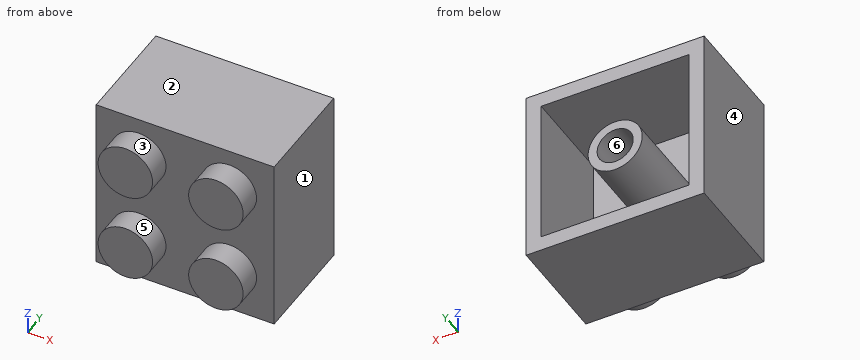
from build123d import *

# Parameters (mm, degrees)
F0_W     = 15.78
F0_H     = 15.78
F0_R     = 2.415
F1_DEPTH = 9.6
F2_DEPTH = 11.76
F3_W     = 13.12
F3_H     = 13.12
F3_R     = 2.415
F3_R_2   = 2.4
F4_DEPTH = 8.38
F3_R_3   = 1.6
F5_DEPTH = 8.38


with BuildPart() as f1:
    # F0 (on Front) → F1 (new body)
    with BuildSketch(Plane.XZ):
        Rectangle(F0_W, F0_H)
        with Locations((-4.115, -3.915)):
            Circle(F0_R, mode=Mode.SUBTRACT)
        with Locations((3.915, -3.915)):
            Circle(F0_R, mode=Mode.SUBTRACT)
        with Locations((-4.115, 4.115)):
            Circle(F0_R, mode=Mode.SUBTRACT)
        with Locations((3.915, 4.115)):
            Circle(F0_R, mode=Mode.SUBTRACT)
    extrude(amount=F1_DEPTH)

    # F0 (on Front) → F2 (join)
    with BuildSketch(Plane.XZ):
        with Locations((-4.115, 4.115)):
            Circle(F0_R)
        with Locations((3.915, 4.115)):
            Circle(F0_R)
        with Locations((-4.115, -3.915)):
            Circle(F0_R)
        with Locations((3.915, -3.915)):
            Circle(F0_R)
    extrude(amount=F2_DEPTH)

    # F3 (on face) → F4 (cut)
    with BuildSketch(Plane.XZ):
        Rectangle(F3_W, F3_H)
        with Locations((-4.115, -3.915)):
            Circle(F3_R, mode=Mode.SUBTRACT)
        with Locations((3.915, -3.915)):
            Circle(F3_R, mode=Mode.SUBTRACT)
        with Locations((-4.115, 4.115)):
            Circle(F3_R, mode=Mode.SUBTRACT)
        Circle(F3_R_2, mode=Mode.SUBTRACT)
        with Locations((3.915, 4.115)):
            Circle(F3_R, mode=Mode.SUBTRACT)
    extrude(amount=F4_DEPTH, mode=Mode.SUBTRACT)

    # F0 (on Front) + F3 (on face) → F5 (cut)
    with BuildSketch(Plane.XZ):
        with Locations((3.915, 4.115)):
            Circle(F0_R)
        with Locations((-4.115, 4.115)):
            Circle(F0_R)
        with Locations((3.915, -3.915)):
            Circle(F0_R)
        with Locations((-4.115, -3.915)):
            Circle(F0_R)
    with BuildSketch(Plane.XZ):
        Circle(F3_R_3)
    extrude(amount=F5_DEPTH, mode=Mode.SUBTRACT)


solid = f1.part
Source: CAD feature listing. Evaluate the final solid. Frame: model axes, mm. Face numbers are marked on the shaded views. A direction names the side the tool comes from. Round coordinates to 2 decimals unless told otherwise and drop trailing zeros. Loops run counter-clockwise (first coordinate to the right, second up) from the corner with the lowest first, then second, coordinate; pieces in that order, holes last.
Q1. First-contact query: P1, Ø6, axis at y = -10, z = -6, coming from the +X side; P2, Ø1, axis at x = -0.5, z = -0.5, coming from the +Y side; P3, Ø3.5, axis at x = 0, z = 0, coming from the -Y side. Flat tips, straight axial feed; report the tip coordinate or a pass-through.
Q2. Access query for the marked faces 4, 5 and 6. Directions: +Z, -Z, +X, -X, +Y, -Y. A direction counts if a zero-diameter tool reaches every point of the face in a straight line with its end or side. Return the directions, or none.
Q3. Section B-B, the plane x = 0. Return loops of the section in (y, z), plus the area to 3 significant figures.
Q4. Mould query, pull axis Z, two halves, no side actions, for the marked faces 1, 2 and 3. Classes: pulls with the +Z half, pulls with the -Z half, needs draft (parallel to the pull), parting line crosses it, or undercut.
Q5. Ray query, line 1 (Z direction, x = 0, y = -2.5); line 2 (Z direction, x = -3.25, y = -4.75). Return the intervals inside material, ascending.
Q6. Section A-A, the plane y = -1.5. Return loops of the section in (x, z).
Q7. Section C-C, the plane z = 0. Return loops of the section in (x, y), plus the area to 3 significant figures.
Solutions:
1. P1: stops at x = 7.89
1. P2: stops at y = -8.38
1. P3: stops at y = -9.6
2. face 4: +Z, -Z, -X, +Y, -Y
2. face 5: -Y
2. face 6: +Y
3. outline: (-9.6, -7.89) - (0, -7.89) - (0, -6.56) - (-8.38, -6.56) - (-8.38, -2.4) - (0, -2.4) - (0, -1.6) - (-8.38, -1.6) - (-8.38, 1.6) - (0, 1.6) - (0, 2.4) - (-8.38, 2.4) - (-8.38, 6.56) - (0, 6.56) - (0, 7.89) - (-9.6, 7.89) - close
3. area: 55.0 mm2
4. face 1: needs draft
4. face 2: pulls with the +Z half
4. face 3: undercut
5. line 1: z = -7.89 to -6.56, -2.4 to -1.6, 1.6 to 2.4, 6.56 to 7.89
5. line 2: z = -7.89 to -6.56, 6.56 to 7.89
6. outline: (-7.89, -7.89) - (7.89, -7.89) - (7.89, 7.89) - (-7.89, 7.89) - close; circle Ø4.8 at (0, 0); hole (-6.56, -6.56) - (6.56, -6.56) - (6.56, 6.56) - (-6.56, 6.56) - close; hole circle Ø3.2 at (0, 0)
7. outline: (-7.89, -9.6) - (7.89, -9.6) - (7.89, 0) - (6.56, 0) - (6.56, -8.38) - (2.4, -8.38) - (2.4, 0) - (1.6, 0) - (1.6, -8.38) - (-1.6, -8.38) - (-1.6, 0) - (-2.4, 0) - (-2.4, -8.38) - (-6.56, -8.38) - (-6.56, 0) - (-7.89, 0) - close
7. area: 55.0 mm2
